Verification items for the finished model (mm, model axes). Face numbers are marked on the shaded views. Round coordinates to 2 decimals unless told otherwise and drop trailing zeros. Write each loop counter-clockwise with the first axis right and the second up, starting at its lowest first coordinate (ties: lowest second). Pieces come first, ordered by that corner, then holes. Notation, with made-up numbers: (58.5, 20) -> (117.5, 20) arc R22 cw to (117.5, 44) -> close; hole circle Ø2 at (27, -27.75). An arc over 180 degrees is marked (long way). Answer as a JSON object with one key per item and string values. Group by question number.
(1) Sectioned sample at A-A on y = 21. Record the cut outline in (x, z).
(2) Gauge pin test, flat ends, axial feed: pin 1 Ø4 at (y, z) = (179, 4.5) entering from -X; pin 2 Ø12 at (y, z) = (157.5, 8.5) entering from +X; pin 3 Ø12 at (x, y) = (9.5, 92.5) entering from -Z. Record the tip position at first contact, or that the pin passes through.
(3) Draft check along Y on the marked faces 1, 2 and 3. Enter one of: released by +Y, released by -Y, zero draft, split by the parting line, or undercut.
(4) Scan lines: L1, parallel to X at y = 68, z = -2.5; L2, parallel to Z at x = -8.5, y = 41.5; L3, parallel to X at y = 81, z = -2.75. Record each from-to range of solid material in increasing order. Write a range as from..to.
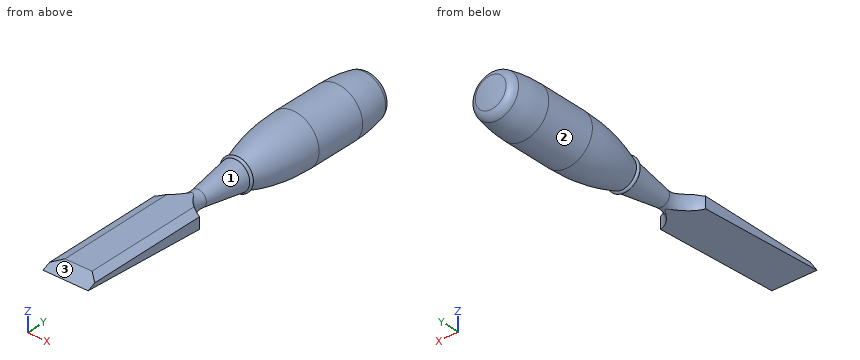
```python
from build123d import *

# Parameters (mm, degrees)
CUT_EXTRUDE1_DEPTH      = 17.51
CUT_EXTRUDE1_DEPTH_BACK = 17.51
SKETCH3_W               = 12.7
SKETCH3_H               = 93.345
CUT_EXTRUDE2_DEPTH      = 15.4780001
CUT_EXTRUDE2_DEPTH_BACK = 15.4780001
CHAMFER1_SIZE           = 1.778
CHAMFER1_SIZE2          = 5.08
CHAMFER1_PART_2_SIZE    = 1.778
CHAMFER1_PART_2_SIZE2   = 5.08


with BuildPart() as part:
    # Sketch1 → Revolve1 (revolve)
    with BuildSketch(Plane.XY):
        with BuildLine():
            Line((0, 0), (0, 200.025))
            ThreePointArc((0, 200.025), (4.361173486, 199.774572862), (8.665015939, 199.026583508))
            ThreePointArc((8.665015939, 199.026583508), (11.099058165, 197.674530854), (12.454800514, 195.242541829))
            ThreePointArc((12.454800514, 195.242541829), (13.970510195, 186.579743755), (14.478, 177.8))
            Line((14.478, 177.8), (14.478, 149.225))
            ThreePointArc((14.478, 149.225), (12.894697981, 130.856561666), (8.1915, 113.03))
            ThreePointArc((8.1915, 113.03), (9.144, 112.0775), (8.1915, 111.125))
            Line((8.1915, 111.125), (4.4958, 86.995))
            ThreePointArc((4.4958, 86.995), (7.228457253, 76.949471101), (16.51, 72.234279615))
            Line((16.51, 72.234279615), (16.51, 0))
            Line((16.51, 0), (0, 0))
        make_face()
    revolve(axis=Axis((0, 0, 0), (0, -1, 0)))

    # Sketch2 → Cut-Extrude1 (cut, two sides)
    with BuildSketch(Plane(origin=(0, 0, 0), x_dir=(0, 0, -1), z_dir=(1, 0, 0))) as cut_extrude1_sk:
        Polygon((4.4958, 86.995), (0, 0), (-3.756857541, 8.509), (-4.4958, 86.995), (-31.75, 86.995), (-31.75, -12.7), (31.75, -12.7), (31.75, 86.995), align=None)
    extrude(amount=CUT_EXTRUDE1_DEPTH, mode=Mode.SUBTRACT)
    extrude(cut_extrude1_sk.sketch, amount=-CUT_EXTRUDE1_DEPTH_BACK, mode=Mode.SUBTRACT)

    # Sketch3 → Cut-Extrude2 (cut, two sides)
    with BuildSketch(Plane.XY) as cut_extrude2_sk:
        with Locations((19.05, 40.3225)):
            Rectangle(SKETCH3_W, SKETCH3_H)
        with Locations((-19.05, 40.3225)):
            Rectangle(SKETCH3_W, SKETCH3_H)
    extrude(amount=CUT_EXTRUDE2_DEPTH, mode=Mode.SUBTRACT)
    extrude(cut_extrude2_sk.sketch, amount=-CUT_EXTRUDE2_DEPTH_BACK, mode=Mode.SUBTRACT)

    # Chamfer1
    chamfer1_edges = [part.edges().sort_by_distance(p)[0] for p in [
        (-12.7, 40.643568714, 4.059403183),
    ]]
    chamfer1_side = [part.faces().sort_by_distance(p)[0] for p in [
        (-12.7, 42.502487943, 0.913030027),
    ]]
    chamfer(chamfer1_edges, length=CHAMFER1_SIZE, length2=CHAMFER1_SIZE2, reference=chamfer1_side[0])

    # Chamfer1 part 2
    chamfer1_part_2_edges = [part.edges().sort_by_distance(p)[0] for p in [
        (12.7, 40.643568715, 4.059403183),
    ]]
    chamfer1_part_2_side = [part.faces().sort_by_distance(p)[0] for p in [
        (12.7, 42.502487941, 0.913030027),
    ]]
    chamfer(chamfer1_part_2_edges, length=CHAMFER1_PART_2_SIZE, length2=CHAMFER1_PART_2_SIZE2, reference=chamfer1_part_2_side[0])


solid = part.part
```
Computed values:
{
 "1": {"outline": "(-12.7, -1.09) -> (12.7, -1.09) -> (12.7, 2.1) -> (7.62, 3.87) -> (-7.62, 3.87) -> (-12.7, 2.1) -> close"},
 "2": {"pin 1": "x = -14.25", "pin 2": "x = 14.26", "pin 3": "z = -4.17"},
 "3": {"face 1": "undercut", "face 2": "zero draft", "face 3": "released by -Y"},
 "4": {"L1": "-12.7..12.7", "L2": "-2.14..3.76", "L3": "-4.18..4.18"}
}
